```python
from build123d import *

# Parameters (mm, degrees)
F0_W     = 26
F0_H     = 26
F1_DEPTH = 4
F2_W     = 5
F2_H     = 26
F3_DEPTH = 3
F4_R     = 2.5
F5_R     = 3
F6_DEPTH = 25
F7_R     = 5.75
F8_DEPTH = 3
F9_SIZE  = 1


with BuildPart() as f1:
    # F0 (on Front) → F1 (new body)
    with BuildSketch(Plane.XZ):
        Rectangle(F0_W, F0_H)
    extrude(amount=-F1_DEPTH)

    # F2 (on face) → F3 (join)
    with BuildSketch(Plane(origin=(0, 4, 0), x_dir=(-1, 0, 0), z_dir=(0, 1, 0))):
        with Locations((4.25, 0)):
            Rectangle(F2_W, F2_H)
    extrude(amount=F3_DEPTH)

    # F4
    f4_edges = [f1.edges().sort_by_distance(p)[0] for p in [
        (-13, 2, 13),
        (-13, 2, -13),
        (13, 2, 13),
        (13, 2, -13),
    ]]
    fillet(f4_edges, radius=F4_R)

    # F5 (on face) → F6 (cut)
    with BuildSketch(Plane.XZ):
        with Locations((5.25, 5.75)):
            Circle(F5_R)
    extrude(amount=-F6_DEPTH, mode=Mode.SUBTRACT)

    # F7 (on face) → F8 (cut)
    with BuildSketch(Plane.XZ):
        with Locations((5.25, 5.75)):
            Circle(F7_R)
    extrude(amount=-F8_DEPTH, mode=Mode.SUBTRACT)

    # F9
    f9_edges = [f1.edges().sort_by_distance(p)[0] for p in [
        (-13, 0, 0),
    ]]
    chamfer(f9_edges, length=F9_SIZE)


solid = f1.part
```
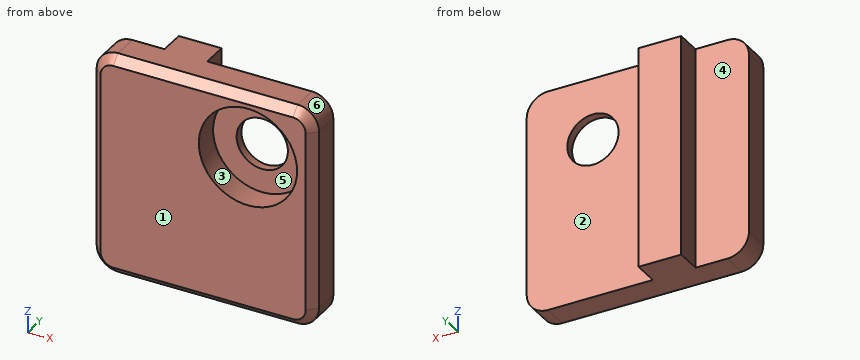
Could you check a few things on this model? Use its own coordinates, in mm. Face numbers are marked on the shaded views. A direction names the side the tool comes from. Coordinates: 2 decimals unless noted, no trailing zeros. Order: outer loops, then holes, each group sorted by start corner. A loop starts at its lowest first (then second) coordinate and runs counter-clockwise, first axis right, second up. Notation, with made-up numbers: M -28.5,26 L -23.5,26 A26 ccw -23.5,61 Z; hole C 7,12 d3. An arc over 180 degrees is marked long. Use a Markdown table: item, result. Add a question column.
Q1. I want a section at D-D on z = -4.5. List the corners of the cut face in (x, y) for me, then the cut area to 3 significant figures.
Q2. I want a section at A-A on z = 5.75. List the corners of the cut face in (x, y) for me, then the cut area to 3 significant figures.
Q3. I want a section at B-B on x = 5.25. List the corners of the cut face in (y, z) for me, then the cut area to 3 significant figures.
Q4. I want a section at C-C on y = 2.5. List the corners of the cut face in (x, z) for me.
Q5. I'm going to push flat-ended pins straight in: pin 1 (3.5 mm diameter, centred on y = 5.5, z = 3.5, fed in from +X); pin 2 (7.5 mm diameter, centred on x = 5, z = 5.5, fed in from +Y); pin 3 (8 mm diameter, centred on x = 5.25, z = 5.75, fed in from -Y); pin 4 (2.5 mm diameter, centred on y = 5.5, z = 4.5, fed in from -X). Where does each tip first touch, or does it pass through?
Q6. Which directions (+Z, -Z, +X, -X, +Y, -Y) give clear straight access to the entire face, cutting with the end or side of a thin tool? Please do the marked faces 1, 2 and 3.
Q7. We'd pull the mould along Z, two halves only. Please class the marked faces 4, 5 and 6: pulls with the +Z half, pulls with the -Z half, needs draft (parallel to the pull), parting line crosses it, or undercut.
Q8. If I drill on L1, parallel to Y at x = 0.25, z = 7.5; L2, parallel to Y at x = -9, z = -6.5; L3, parallel to Z at x = 5.25, y = 3.7, over which ranges is the centre line in solid material (lowest first)?
Checked values:
| question | item | result |
|---|---|---|
| 1 | outline | M -13,1 L -12,0 L 12,0 L 13,1 L 13,4 L -1.75,4 L -1.75,7 L -6.75,7 L -6.75,4 L -13,4 Z |
| 1 | area | 118 mm² |
| 2 | outline | M -13,1 L -12,0 L -0.5,0 L -0.5,3 L 2.25,3 L 2.25,4 L -1.75,4 L -1.75,7 L -6.75,7 L -6.75,4 L -13,4 Z; M 8.25,3 L 11,3 L 11,0 L 12,0 L 13,1 L 13,4 L 8.25,4 Z |
| 2 | area | 77.5 mm² |
| 3 | outline | M 0,-12 L 1,-13 L 4,-13 L 4,2.75 L 3,2.75 L 3,0 L 0,0 Z; M 0,11.5 L 3,11.5 L 3,8.75 L 4,8.75 L 4,13 L 1,13 L 0,12 Z |
| 3 | area | 62.5 mm² |
| 4 | outline | M -13,-10.5 A2.5 ccw -10.5,-13 L 10.5,-13 A2.5 ccw 13,-10.5 L 13,10.5 A2.5 ccw 10.5,13 L -10.5,13 A2.5 ccw -13,10.5 Z; hole C 5.25,5.75 d11.5 |
| 5 | pin 1 | x = 13 |
| 5 | pin 2 | y = 4 |
| 5 | pin 3 | y = 3 |
| 5 | pin 4 | x = -6.75 |
| 6 | face 1 | +Z, -Z, +X, -X, -Y |
| 6 | face 2 | +Z, -Z, +X, +Y |
| 6 | face 3 | -Y |
| 7 | face 4 | needs draft |
| 7 | face 5 | undercut |
| 7 | face 6 | pulls with the +Z half |
| 8 | L1 | 3 to 4 |
| 8 | L2 | 0 to 4 |
| 8 | L3 | -13 to 2.75, 8.75 to 13 |
